Study the drawing (mm; zero at the part's minimum x, y, z) and answer. A direction names the side the tool comes from. Give positions to 0.01 mm unless a question says otherwise; leave off trailing zeros. Write each loop counter-clockwise with the first axis right and the second up, starting at its lowest first coordinate (ties: lowest second). Pieces come first, ordered by that corner, then holes. Notation, with made-up numbers: (-12.5, -15) - (34.5, -15) arc R29 cw to (34.5, 15) - close; hole circle Ø5 at (-36.5, -22.5). An arc over 180 degrees is marked (long way). Answer in a Markdown table with one row per item. Add a question column.
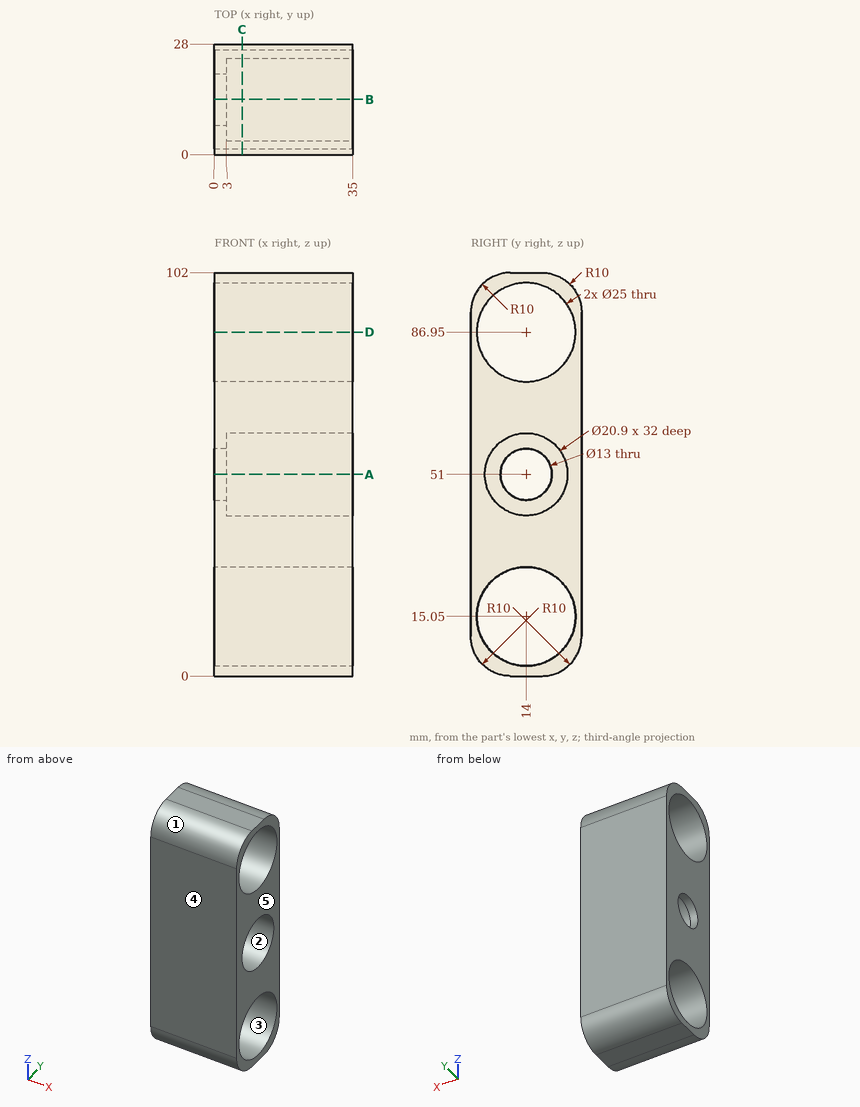
1. A tool of negligible diameter and unlimited length cuts with its end or side. For the marked faces 1 and 2, from which of +Z, -Z, +X, -X, +Y, -Y can it reach the whole face along a straight path? Write none if from no direction.
2. Section C-C (x = 7) is taken. Give the vertices of the cut face in (y, z), and give its area (3 significant figures).
3. Given pin 1 Ø4 at (x, y) = (25.5, 4) entering from -Z; pin 2 Ø8 at (y, z) = (18, 47) entering from +X, each flat-ended and moving along its own axis, determine where each tip first touches the part or whether it passes through.
4. The mould has two halves that part along Y. Classify the marked faces 3, 4 and 5: +Y half, -Y half, draft (parallel to the pull), parting line (faces both ways), or undercut.
5. Section D-D (z = 86.95) is taken. Give the vertices of the cut face in (x, y).
6. Section A-A (z = 51) is taken. Give the vertices of the cut face in (x, y), and give its area (3 significant figures).
7. Section B-B (y = 14) is taken. Give the vertices of the cut face in (x, z), and give its area (3 significant figures).
8. Straight lines are drawn through the part: L1, parallel to Y at x = 18, z = 86.95; L2, parallel to Y at x = 17, z = 51; L3, parallel to Z at x = 18.5, y = 10.75. For each, find the intervals that lie inside material, in ascending order. Write a range as [from, to].
Geometry check:
| question | item | result |
|---|---|---|
| 1 | face 1 | +Z, +X, -X, -Y |
| 1 | face 2 | +X |
| 2 | outline | (0, 10) arc R10 ccw to (10, 0) - (18, 0) arc R10 ccw to (28, 10) - (28, 92) arc R10 ccw to (18, 102) - (10, 102) arc R10 ccw to (0, 92) - close; hole circle Ø25 at (14, 15.05); hole circle Ø25 at (14, 86.95); hole circle Ø20.9 at (14, 51) |
| 2 | area | 1,450 mm² |
| 3 | pin 1 | z = 0.83 |
| 3 | pin 2 | x = 3 |
| 4 | face 3 | undercut |
| 4 | face 4 | -Y half |
| 4 | face 5 | draft |
| 5 | outline | (0, 0) - (35, 0) - (35, 1.5) - (0, 1.5) - close; (0, 26.5) - (35, 26.5) - (35, 28) - (0, 28) - close |
| 6 | outline | (0, 0) - (35, 0) - (35, 3.55) - (3, 3.55) - (3, 7.5) - (0, 7.5) - close; (0, 20.5) - (3, 20.5) - (3, 24.45) - (35, 24.45) - (35, 28) - (0, 28) - close |
| 6 | area | 272 mm² |
| 7 | outline | (0, 0) - (35, 0) - (35, 2.55) - (0, 2.55) - close; (0, 27.55) - (35, 27.55) - (35, 40.55) - (3, 40.55) - (3, 44.5) - (0, 44.5) - close; (0, 57.5) - (3, 57.5) - (3, 61.45) - (35, 61.45) - (35, 74.45) - (0, 74.45) - close; (0, 99.45) - (35, 99.45) - (35, 102) - (0, 102) - close |
| 7 | area | 1,110 mm² |
| 8 | L1 | [0, 1.5], [26.5, 28] |
| 8 | L2 | [0, 3.55], [24.45, 28] |
| 8 | L3 | [0, 2.98], [27.12, 41.07], [60.93, 74.88], [99.02, 102] |
